The model under review builds one solid part; all positions refer to its coordinate system, in mm. A direction names the side the tool comes from. Round coordinates to 2 decimals unless told otherwise and drop trailing zeros. Write each loop counter-clockwise with the first axis right and the second up, starting at its lowest first coordinate (ties: lowest second). Pieces come first, ordered by that corner, then holes. Notation, with made-up numbers: (2, 62) - (28, 62) arc R24 ccw to (28, 85) - close; hole circle Ø7 at (-37, 70.5). An arc over 180 degrees is marked (long way). Use one line per item in the form item = value.
from build123d import *

# Parameters (mm, degrees)
SKETCH_1_R      = 2.75
EXTRUDE_1_DEPTH = 3
SKETCH_2_R      = 1.5
EXTRUDE_2_DEPTH = 10
EXTRUDE_3_DEPTH = 1


with BuildPart() as part:
    # Sketch 1 → Extrude 1 (new body)
    with BuildSketch(Plane.XY):
        Circle(SKETCH_1_R)
        Polygon((1.732050808, 0), (0.866025404, 1.5), (-0.866025404, 1.5), (-1.732050808, 0), (-0.866025404, -1.5), (0.866025404, -1.5), align=None, mode=Mode.SUBTRACT)
    extrude(amount=EXTRUDE_1_DEPTH)



with BuildPart() as body_2:
    # Sketch 2 → Extrude 2 (new body)
    with BuildSketch(Plane(origin=(0, 0, 0), x_dir=(-1, 0, 0), z_dir=(0, 0, -1))):
        Circle(SKETCH_2_R)
    extrude(amount=EXTRUDE_2_DEPTH)


with BuildPart() as part_1:
    add(part.part)

    add(body_2.part)  # Extrude 3 merges body 2
    # Sketch 1_3 → Extrude 3 (add)
    with BuildSketch(Plane.XY):
        Polygon((-0.866025404, -1.5), (0.866025404, -1.5), (1.732050808, 0), (0.866025404, 1.5), (-0.866025404, 1.5), (-1.732050808, 0), align=None)
    extrude(amount=EXTRUDE_3_DEPTH)


solid = part_1.part
(1) Add section A-A on x = 0. Write out the cut boundary in (y, z).
Geometry results:
outline = (-2.75, 0) - (-1.5, 0) - (-1.5, -10) - (1.5, -10) - (1.5, 0) - (2.75, 0) - (2.75, 3) - (1.5, 3) - (1.5, 1) - (-1.5, 1) - (-1.5, 3) - (-2.75, 3) - close
(2) The part is to be moulded in two halves that separate along Y. For faces 4 (the flat face through (0, 0, -10)), 5 (the flat face through (1.305, 0.74, 1.986)), 6 (the flat face through (1.293, -0.76, 1.986)), 7 (the cylindrical face through (1.5, 0.07, -4.93)), say which applies: +Y half, -Y half, draft (parallel to the pull), parting line (faces both ways), or undercut.
Geometry results:
face_4 = draft
face_5 = undercut
face_6 = undercut
face_7 = parting line
(3) Add section C-C on z = 0.5. Write out the cut boundary in (x, y), then the cut area to 3 significant figures.
Geometry results:
outline = circle Ø5.5 at (0, 0)
area = 23.8 mm2
(4) Insertion check: P1, Ø0.5, axis at x = -0.5, z = 2.5, coming from the +Y side; P2, Ø1, axis at x = 0, y = 0, coming from the +Z side; P3, Ø1.5, axis at x = -2, z = -2.5, coming from the +Y side. Each pin has a flat end and moves straight along its axis. Give the tip position at first contact, or say it passes through.
Geometry results:
P1 = 2.74
P2 = 1
P3 = 0.83
(5) To check wall thickness, follow L1, parallel to Z at x = 1.2, y = 0; L2, parallel to Z at x = -0.3, y = -2.3; L3, parallel to X at y = -1, z = 1.5. State the ranges of each line that lie inside material, in increasing order.
Geometry results:
L1 = -10 to 1
L2 = 0 to 3
L3 = -2.56 to -1.15, 1.15 to 2.56
(6) Machinability: for faces 1 (the flat face through (2, 0, 3)), 2 (the flat face through (0, -1.5, 2)), 3 (the flat face through (1.2, -1.2, 0)), which of the approach directions +Z, -Z, +X, -X, +Y, -Y give a long, thin tool a straight path to every point of the face, cutting with its end or side? Answer none if there is none.
Geometry results:
face_1 = +Z, +X, -X, +Y, -Y
face_2 = +Z
face_3 = -Z
(7) Add section B-B on y = -0.35. Write out the cut boundary in (x, z), then the cut area to 3 significant figures.
Geometry results:
outline = (-2.73, 0) - (-1.46, 0) - (-1.46, -10) - (1.46, -10) - (1.46, 0) - (2.73, 0) - (2.73, 3) - (1.53, 3) - (1.53, 1) - (-1.53, 1) - (-1.53, 3) - (-2.73, 3) - close
area = 39.4 mm2
(8) Add section D-D on z = -6. Write out the cut boundary in (x, y), then the cut area to 3 significant figures.
Geometry results:
outline = circle Ø3 at (0, 0)
area = 7.07 mm2
